Input: part model. Units: mm. Frame: model coordinates. Round coordinates to 2 decimals unless told otherwise and drop trailing zeros. Loops run counter-clockwise (first coordinate to the right, second up) from the corner with the lowest first, then second, coordinate; pieces in that order, holes last.
(1) Line query: line 1 (Y direction, x = -67, z = 3.55); line 2 (X direction, y = 127, z = 0.6); line 3 (X direction, y = 134, z = 2.6). Output: solid intervals per line, ascending.
(2) Cut plane B-B, the plane x = -51. Output: boundary loops of the cut face in (y, z).
(3) Cut plane A-A, the plane z = 0.8. Give the number of separate pieces and of enclosed holes in the cut face, and give its area (3 significant figures).
(4) First-contact query: pin 1 Ø10 at (x, y) = (-72, 175.5) entering from -Z; pin 2 Ø3 at (x, y) = (-176.5, 134) entering from +Z. Flat tips, straight axial feed; report the tip coordinate or a pass-through.
from build123d import *

# Parameters (mm, degrees)
ESQUISSE1_W        = 5
ESQUISSE1_H        = 5
ESQUISSE1_R        = 2
ESQUISSE1_W_2      = 40
ESQUISSE1_H_2      = 140
BOSS_EXTRU_1_DEPTH = 5
CONG_1_R           = 10


with BuildPart() as part:
    # Esquisse1 → Boss.-Extru.1 (new body)
    with BuildSketch(Plane.XY):
        Polygon((-182, 196), (-182, 188), (-182, 0), (-182, -8), (48, -8), (48, 0), (48, 188), (48, 196), align=None)
        with Locations((-144.5, -2.5)):
            Rectangle(ESQUISSE1_W, ESQUISSE1_H, mode=Mode.SUBTRACT)
        with Locations((-137, -2.5)):
            Circle(ESQUISSE1_R, mode=Mode.SUBTRACT)
        with Locations((-129.5, -2.5)):
            Rectangle(ESQUISSE1_W, ESQUISSE1_H, mode=Mode.SUBTRACT)
        with Locations((-74.5, -2.5)):
            Rectangle(ESQUISSE1_W, ESQUISSE1_H, mode=Mode.SUBTRACT)
        with Locations((-67, -2.5)):
            Circle(ESQUISSE1_R, mode=Mode.SUBTRACT)
        with Locations((-59.5, -2.5)):
            Rectangle(ESQUISSE1_W, ESQUISSE1_H, mode=Mode.SUBTRACT)
        with Locations((-4.5, -2.5)):
            Rectangle(ESQUISSE1_W, ESQUISSE1_H, mode=Mode.SUBTRACT)
        with Locations((3, -2.5)):
            Circle(ESQUISSE1_R, mode=Mode.SUBTRACT)
        with Locations((10.5, -2.5)):
            Rectangle(ESQUISSE1_W, ESQUISSE1_H, mode=Mode.SUBTRACT)
        with Locations((-176.5, 46.5)):
            Rectangle(ESQUISSE1_W, ESQUISSE1_H, mode=Mode.SUBTRACT)
        with Locations((-176.5, 54)):
            Circle(ESQUISSE1_R, mode=Mode.SUBTRACT)
        with Locations((-176.5, 61.5)):
            Rectangle(ESQUISSE1_W, ESQUISSE1_H, mode=Mode.SUBTRACT)
        with Locations((-134, 94)):
            Rectangle(ESQUISSE1_W_2, ESQUISSE1_H_2, mode=Mode.SUBTRACT)
        with Locations((-176.5, 126.5)):
            Rectangle(ESQUISSE1_W, ESQUISSE1_H, mode=Mode.SUBTRACT)
        with Locations((-176.5, 134)):
            Circle(ESQUISSE1_R, mode=Mode.SUBTRACT)
        with Locations((-176.5, 141.5)):
            Rectangle(ESQUISSE1_W, ESQUISSE1_H, mode=Mode.SUBTRACT)
        with Locations((-144.5, 190.5)):
            Rectangle(ESQUISSE1_W, ESQUISSE1_H, mode=Mode.SUBTRACT)
        with Locations((-137, 190.5)):
            Circle(ESQUISSE1_R, mode=Mode.SUBTRACT)
        with Locations((-129.5, 190.5)):
            Rectangle(ESQUISSE1_W, ESQUISSE1_H, mode=Mode.SUBTRACT)
        with Locations((-74.5, 190.5)):
            Rectangle(ESQUISSE1_W, ESQUISSE1_H, mode=Mode.SUBTRACT)
        Polygon((-89, 125.5), (-45, 125.5), (-45, 50.5), (-67, 50.5), (-89, 50.5), align=None, mode=Mode.SUBTRACT)
        with Locations((42.5, 46.5)):
            Rectangle(ESQUISSE1_W, ESQUISSE1_H, mode=Mode.SUBTRACT)
        with Locations((0, 94)):
            Rectangle(ESQUISSE1_W_2, ESQUISSE1_H_2, mode=Mode.SUBTRACT)
        with Locations((42.5, 54)):
            Circle(ESQUISSE1_R, mode=Mode.SUBTRACT)
        with Locations((42.5, 61.5)):
            Rectangle(ESQUISSE1_W, ESQUISSE1_H, mode=Mode.SUBTRACT)
        with Locations((-67, 190.5)):
            Circle(ESQUISSE1_R, mode=Mode.SUBTRACT)
        with Locations((-59.5, 190.5)):
            Rectangle(ESQUISSE1_W, ESQUISSE1_H, mode=Mode.SUBTRACT)
        with Locations((42.5, 126.5)):
            Rectangle(ESQUISSE1_W, ESQUISSE1_H, mode=Mode.SUBTRACT)
        with Locations((42.5, 134)):
            Circle(ESQUISSE1_R, mode=Mode.SUBTRACT)
        with Locations((42.5, 141.5)):
            Rectangle(ESQUISSE1_W, ESQUISSE1_H, mode=Mode.SUBTRACT)
        with Locations((-4.5, 190.5)):
            Rectangle(ESQUISSE1_W, ESQUISSE1_H, mode=Mode.SUBTRACT)
        with Locations((3, 190.5)):
            Circle(ESQUISSE1_R, mode=Mode.SUBTRACT)
        with Locations((10.5, 190.5)):
            Rectangle(ESQUISSE1_W, ESQUISSE1_H, mode=Mode.SUBTRACT)
    extrude(amount=BOSS_EXTRU_1_DEPTH)

    # Congé1
    cong_1_edges = [part.edges().sort_by_distance(p)[0] for p in [
        (-154, 24, 2.5),
        (-114, 24, 2.5),
        (-114, 164, 2.5),
        (-154, 164, 2.5),
        (-20, 164, 2.5),
        (-20, 24, 2.5),
        (20, 24, 2.5),
        (20, 164, 2.5),
        (-45, 125.5, 2.5),
        (-89, 125.5, 2.5),
        (-89, 50.5, 2.5),
        (-45, 50.5, 2.5),
    ]]
    fillet(cong_1_edges, radius=CONG_1_R)


solid = part.part
Reported:
1. line 1: y = -8 to -4.5, -0.5 to 50.5, 125.5 to 188.5, 192.5 to 196
1. line 2: x = -182 to -179, -174 to -154, -114 to -20, 20 to 40, 45 to 48
1. line 3: x = -182 to -178.5, -174.5 to -154, -114 to -20, 20 to 40.5, 44.5 to 48
2. outline: (-8, 0) - (51.33, 0) - (51.33, 5) - (-8, 5) - close; (124.67, 0) - (196, 0) - (196, 5) - (124.67, 5) - close
3. separate pieces: 1
3. enclosed holes: 33
3. area: 32,100 mm2
4. pin 1: stops at z = 0
4. pin 2: passes through
